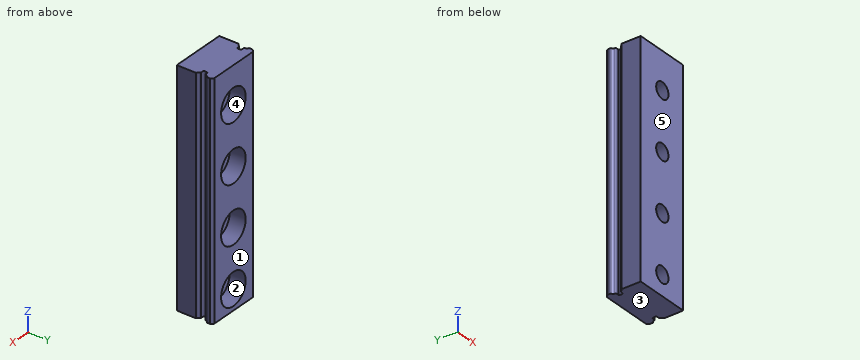
Autodesk Inventor part; units mm, degrees
ref_plane "YZ Plane" through (0, 0, 0) normal (1, 0, 0) x (0, 1, 0)
ref_plane "XZ Plane" through (0, 0, 0) normal (0, 1, 0) x (-1, 0, 0)
ref_plane "XY Plane" through (0, 0, 0) normal (0, 0, 1) x (1, 0, 0)
ref_plane "Work Plane1" through (0, 0, 0) normal (0, 0, 1) x (1, 0, 0)
sketch "Sketch1" plane through (0, 0, 0) normal (0, 0, 1) x (1, 0, 0)
  line L0 (0, 0) -> (5.55, 0)
  line L1 (6.05, -7.8) -> (0, -7.8)
  line L2 (0, -7.8) -> (0, 0)
  line L3 (5.55, 0) -> (6.05, -0.5)
  arc A0 (6.05, -3.6294) -> (5.8482, -3.4873) centre (5.8013, -3.7683) ccw
  arc A1 (5.5514, -3.0941) -> (5.8482, -3.4873) centre (6.6343, -2.5853) ccw
  arc A2 (5.5514, -3.0941) -> (5.425, -2.9829) centre (5.3332, -3.2146) ccw
  line L4 (5.425, -2.9829) -> (4.928, -2.9441)
  arc A3 (4.7, -2.7255) -> (4.928, -2.9441) centre (4.9475, -2.6956) ccw
  arc A4 (4.9275, -2.0261) -> (4.7, -2.2744) centre (4.9493, -2.2744) ccw
  arc A5 (5.293, -1.9942) -> (5.5514, -1.8412) centre (5.3208, -1.7464) ccw
  arc A6 (5.8954, -1.3233) -> (5.5514, -1.8412) centre (6.7024, -2.2326) ccw
  arc A7 (5.8954, -1.3233) -> (6.05, -1.1) centre (5.8008, -1.0927) ccw
  line L5 (5.293, -1.9942) -> (4.9275, -2.0261)
  line L6 (4.7, -2.7255) -> (4.7, -2.2744)
  line L7 (6.05, -0.5) -> (6.05, -1.1)
  line L8 (6.05, -3.6294) -> (6.05, -7.8)
  point P0 (6.05, 0)
  dimension "d0" = 0.5
  dimension "d1" = 0.5
  dimension "d17" = 6.05
  dimension "d18" = 7.8
  dimension "d20" = 2.6756
  dimension "d21" = 0.5
  dimension "d22" = 1.1
  dimension "d23" = 4.7
  dimension "d24" = 0.2275
  dimension "d25" = 0.228
  dimension "d26" = 0
  dimension "d27" = 0.2483
  dimension "d28" = 0.2186
extrude "Extrusion1" add sketch "Sketch1" along normal blind 50
mirror "Mirror1" about plane through (0, 0, 0) normal (-1, 0, 0) of "Extrusion1"
sketch "Sketch2" plane through (5.55, 0, 50) normal (0, 1, 0) x (1, 0, 0)
  line L0 (-11.1, 50) -> (0, 50)
  line L1 (-11.1, 50) -> (-11.1, 0)
  line L2 (0, 0) -> (-11.1, 0)
  line L3 (0, 50) -> (0, 0)
  point P0 (-5.55, 50)
  point P1 (-5.45, 45.5983)
hole "Hole1" at (0.1, 0, 4.4017) direction (0, -1, 0) diameter 3.5 end through all counterbore diameter 7 counterbore depth 3.5
pattern_linear "Rectangular Pattern1" count 5 spacing 12.5 along (0, 0, 1) of "Hole1"
ref_plane "Work Plane2" through (0, -7.8, 0) normal (1, 0, 0) x (0, 0, -1)
ref_plane "Arbeitsebene3" through (0, 0, 25) normal (0, 0, 1) x (1, 0, 0)
properties part number "30_Cube_Z_Focus_MGN_NEMA_rail"
Could you check a few things on this model? Use its own coordinates, in mm. Face numbers are marked on the shaded views. A direction names the side the tool comes from. Coordinates: 2 decimals unless noted, no trailing zeros. Loops run counter-clockwise (first coordinate to the right, second up) from the corner with the lowest first, then second, coordinate; pieces in that order, holes last.
1) Imagine slicing it at A-A (y = -5). List the corners of the cut face in (x, z) for me, and give its area (3 significant figures).
Reported:
outline: (-6.05, 0) - (6.05, 0) - (6.05, 50) - (-6.05, 50) - close; hole circle Ø3.5 at (0.1, 4.4); hole circle Ø3.5 at (0.1, 16.9); hole circle Ø3.5 at (0.1, 29.4); hole circle Ø3.5 at (0.1, 41.9)
area: 567 mm2
2) Will this pin go through, and if not, where does the flat tip stop? pin 1 Ø4.5 at (x, z) = (0.1, 16.9) entering from +Y.
Reported:
pin 1: stops at y = -3.5
3) Imagine slicing it at B-B (x = 0.1). State how many separate pieces and enclosed holes the cut face has, and give its area (3 significant figures).
Reported:
separate pieces: 5
enclosed holes: 0
area: 232 mm2
4) Which directions (+Z, -Z, +X, -X, +Y, -Y) give clear straight access to the entire face, cutting with the end or side of a thin tool? Please do the marked faces 4 and 5.
Reported:
face 4: +Y
face 5: +Z, -Z, +X, -X, -Y
5) Thinking about a two-plate mould opening in Z: for the marked faces 1, 2 and 3, which applies, released by +Z, released by -Z, zero draft, split by the parting line, or undercut?
Reported:
face 1: zero draft
face 2: undercut
face 3: released by -Z
6) Please list where these lines run through material, in increasing order: line 1 along Z through (x, y) = (0.1, -2.5); line 2 along Z through (x, y) = (0.1, -4.95); line 3 along X through (y, z) = (-2.25, 42).
Reported:
line 1: z = 0 to 0.9, 7.9 to 13.4, 20.4 to 25.9, 32.9 to 38.4, 45.4 to 50
line 2: z = 0 to 2.65, 6.15 to 15.15, 18.65 to 27.65, 31.15 to 40.15, 43.65 to 50
line 3: x = -4.7 to -3.4, 3.6 to 4.7
7) Imagine slicing it at D-D (x = -2.5). List the corners of the cut face in (y, z) for me.
Reported:
outline: (-7.8, 0) - (0, 0) - (0, 2.06) - (-3.5, 2.06) - (-3.5, 6.74) - (0, 6.74) - (0, 14.56) - (-3.5, 14.56) - (-3.5, 19.24) - (0, 19.24) - (0, 27.06) - (-3.5, 27.06) - (-3.5, 31.74) - (0, 31.74) - (0, 39.56) - (-3.5, 39.56) - (-3.5, 44.24) - (0, 44.24) - (0, 50) - (-7.8, 50) - close
